Geometry: final body of the model. Coordinates: model frame, mm. A direction names the side the tool comes from. Give positions to 0.01 mm unless a question says otherwise; leave off trailing zeros. Order: outer loops, then holes, each group sorted by start corner. A loop starts at its lowest first (then second) coordinate and runs counter-clockwise, first axis right, second up. Notation, with made-up numbers: (45, 44.5) -> (99, 44.5) arc R7 ccw to (99, 50.5) -> close; hole circle Ø10 at (0.5, 57.5). An arc over 180 degrees is marked (long way). One line per question, with ' | ' between items.
from build123d import *

# Parameters (mm, degrees)
F1_DEPTH = 25.4
F3_DEPTH = 12.701
F5_DEPTH = 9.9016336957


with BuildPart() as f1:
    # F0 (on Front) → F1 (new body)
    with BuildSketch(Plane.XZ):
        Polygon((-29.7019003412, 0), (27.4480996588, 0), (27.4480996588, 9.9006336957), (-17.0019003412, 9.9006336957), (-17.0019003412, 27.2871126172), (-29.7019003412, 27.2871126172), align=None)
    extrude(amount=F1_DEPTH)

    # F2 (on face) → F3 (cut, through all)
    with BuildSketch(Plane.YZ.offset(-17.0019003412)):
        with BuildLine():
            Line((-25.4, 27.2871126172), (-25.4, 18.5938731565))
            ThreePointArc((-25.4, 18.5938731565), (-22.9225497247, 23.7099564427), (-18.5048555567, 27.2871126172))
            Line((-18.5048555567, 27.2871126172), (-25.4, 27.2871126172))
        make_face()
        with BuildLine():
            ThreePointArc((-7.2696510886, 18.5938731565), (-12.7, 24.0242220678), (-18.1303489114, 18.5938731565))
            Line((-18.1303489114, 18.5938731565), (-7.2696510886, 18.5938731565))
        make_face()
        with BuildLine():
            Line((-18.1303489114, 27.2871126172), (-18.1303489114, 18.5938731565))
            ThreePointArc((-18.1303489114, 18.5938731565), (-12.7, 24.0242220678), (-7.2696510886, 18.5938731565))
            Line((-7.2696510886, 18.5938731565), (-7.2696510886, 27.2871126172))
            Line((-7.2696510886, 27.2871126172), (-18.1303489114, 27.2871126172))
        make_face()
        with BuildLine():
            Line((-7.2696510886, 18.5938731565), (-18.1303489114, 18.5938731565))
            ThreePointArc((-18.1303489114, 18.5938731565), (-12.7, 13.1635242451), (-7.2696510886, 18.5938731565))
        make_face()
        with BuildLine():
            ThreePointArc((-6.8951444433, 27.2871126172), (-12.7, 28.6495177359), (-18.5048555567, 27.2871126172))
            Line((-18.5048555567, 27.2871126172), (-18.1303489114, 27.2871126172))
            Line((-18.1303489114, 27.2871126172), (-7.2696510886, 27.2871126172))
            Line((-7.2696510886, 27.2871126172), (-6.8951444433, 27.2871126172))
        make_face()
        with BuildLine():
            Line((0, 27.2871126172), (-6.8951444433, 27.2871126172))
            ThreePointArc((-6.8951444433, 27.2871126172), (-2.4774502753, 23.7099564427), (0, 18.5938731565))
            Line((0, 18.5938731565), (0, 27.2871126172))
        make_face()
    extrude(amount=-F3_DEPTH, mode=Mode.SUBTRACT)

    # F4 (on face) → F5 (cut, through all)
    with BuildSketch(Plane.XY.offset(9.9006336957)):
        with BuildLine():
            Line((14.7480996588, -19.05), (14.7480996588, -6.35))
            ThreePointArc((14.7480996588, -6.35), (8.3980996588, -12.7), (14.7480996588, -19.05))
        make_face()
        with BuildLine():
            ThreePointArc((21.0980996588, -12.7), (19.2382277193, -8.2098719395), (14.7480996588, -6.35))
            Line((14.7480996588, -6.35), (14.7480996588, -19.05))
            ThreePointArc((14.7480996588, -19.05), (19.2382277193, -17.1901280605), (21.0980996588, -12.7))
        make_face()
        with BuildLine():
            Line((-4.3019003412, -19.05), (-4.3019003412, -6.35))
            ThreePointArc((-4.3019003412, -6.35), (-10.6519003412, -12.7), (-4.3019003412, -19.05))
        make_face()
        with BuildLine():
            ThreePointArc((2.0480996588, -12.7), (0.1882277193, -8.2098719395), (-4.3019003412, -6.35))
            Line((-4.3019003412, -6.35), (-4.3019003412, -19.05))
            ThreePointArc((-4.3019003412, -19.05), (0.1882277193, -17.1901280605), (2.0480996588, -12.7))
        make_face()
        with BuildLine():
            Line((27.4480996588, 0), (14.7480996588, 0))
            ThreePointArc((14.7480996588, 0), (23.7283557799, -3.7197438789), (27.4480996588, -12.7))
            Line((27.4480996588, -12.7), (27.4480996588, 0))
        make_face()
        with BuildLine():
            Line((27.4480996588, -25.4), (27.4480996588, -12.7))
            ThreePointArc((27.4480996588, -12.7), (23.7283557799, -21.6802561211), (14.7480996588, -25.4))
            Line((14.7480996588, -25.4), (27.4480996588, -25.4))
        make_face()
    extrude(amount=-F5_DEPTH, mode=Mode.SUBTRACT)


solid = f1.part
1) Section C-C on z = 25. Return loops of the section in (x, y), plus the area to 3 significant figures.
Check result:
outline: (-29.7, -21.75) -> (-17, -21.75) -> (-17, -18.13) -> (-29.7, -18.13) -> close; (-29.7, -7.27) -> (-17, -7.27) -> (-17, -3.65) -> (-29.7, -3.65) -> close | area: 92.0 mm^2
2) Contact query for flat-ended pins moving along their axis: pin 1 Ø2.5 at (x, z) = (-25, 21.5) entering from -Y; pin 2 Ø3 at (x, y) = (19.5, -15) entering from +Z; pin 3 Ø5 at (y, z) = (-9.5, 16) entering from +X. Output: stop coordinate, or through.
Check result:
pin 1: stops at y = -24.89 | pin 2: stops at z = 9.9 | pin 3: stops at x = -17
3) Section A-A on x = 20.5. Return loops of the section in (y, z), plus the area to 3 significant figures.
Check result:
outline: (-24.02, 0) -> (-15.39, 0) -> (-15.39, 9.9) -> (-24.02, 9.9) -> close; (-10.01, 0) -> (-1.38, 0) -> (-1.38, 9.9) -> (-10.01, 9.9) -> close | area: 171 mm^2
4) Pull-direction query (Y, two-part tool) for faces 1 (the flat face through (-23, -7.27, 23)), 2 (the flat face through (-13, 0, 7)), 3 (the flat face through (6, -13, 9.901)); classes: +Y half, -Y half, draft (parallel to the pull), parting line (faces both ways), or undercut.
Check result:
face 1: undercut | face 2: +Y half | face 3: draft
5) Section B-B on y = -10.25. Return loops of the section in (x, z), plus the area to 3 significant figures.
Check result:
outline: (-29.7, 0) -> (-10.16, 0) -> (-10.16, 9.9) -> (-17, 9.9) -> (-17, 13.75) -> (-29.7, 13.75) -> close; (1.56, 0) -> (8.89, 0) -> (8.89, 9.9) -> (1.56, 9.9) -> close; (20.61, 0) -> (27.21, 0) -> (27.21, 9.9) -> (20.61, 9.9) -> close | area: 380 mm^2
6) Section D-D on z = 6.75. Return loops of the section in (x, y).
Check result:
outline: (-29.7, -25.4) -> (14.75, -25.4) arc R12.7 ccw to (14.75, 0) -> (-29.7, 0) -> close; hole circle Ø12.7 at (-4.3, -12.7); hole circle Ø12.7 at (14.75, -12.7)
7) Set-up query: faces 4 (the flat face through (-23, -18.13, 23)), 5 (the flat face through (-17.002, -13, 13)), 6 (the flat face through (-29.702, -13, 11)). Return all of +Z, -Z, +X, -X, +Y, -Y with unobstructed straight access to the full face (end or side cutting, diameter ignored); none if empty.
Check result:
face 4: +Z, +X, -X | face 5: +Z, +X, +Y, -Y | face 6: +Z, -Z, -X, +Y, -Y
8) Material intervals for probe 1 along X at (y, z) = (-12.75, 6); probe 2 along X at (y, z) = (-10.5, 2); probe 3 along X at (y, z) = (-16.5, 11.5), sorted ascending. Write a range as from..to.
Check result:
probe 1: x = -29.7..-10.65, 2.05..8.4, 21.1..27.45 | probe 2: x = -29.7..-10.26, 1.65..8.79, 20.7..27.26 | probe 3: x = -29.7..-17
